Answer from the drawing. Dimensions are ordinates in mm from the lowest x, y and z of the part. A direction names the side the tool comes from. Give positions to 0.01 mm unless a question says otherwise; leave off trailing zeros. Order: outer loops, then holes, each group sorted by start corner. A loop starts at its lowest first (then second) coordinate and runs counter-clockwise, first axis right, second up.
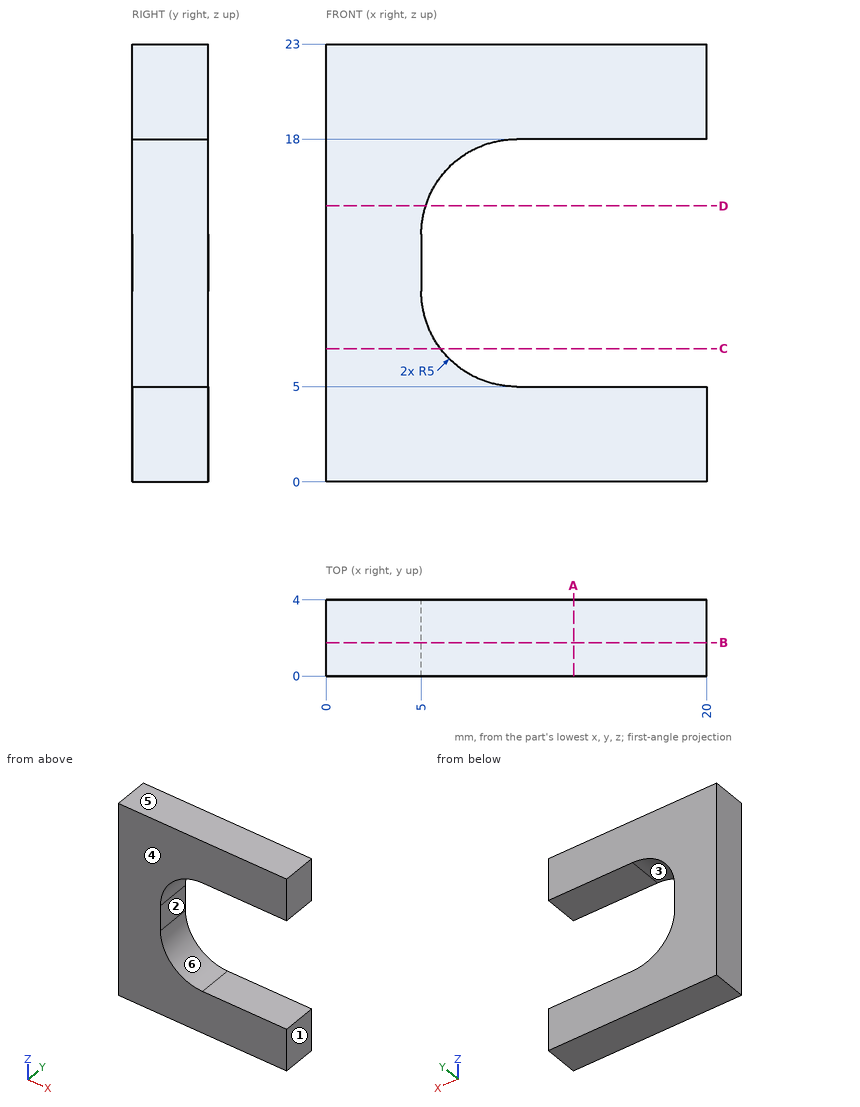
1. The mould has two halves that part along Z. Classify the marked faces 3, 4, 5 and 6: pulls with the +Z half, pulls with the -Z half, needs draft (parallel to the pull), parting line crosses it, or undercut.
Findings below:
face 3: undercut
face 4: needs draft
face 5: pulls with the +Z half
face 6: undercut
2. The part is cut by section B-B (y = 1.75). Write down the section's boundary in (x, z).
Findings below:
outline: (0, 0) - (20, 0) - (20, 5) - (10, 5) arc R5 cw to (5, 10) - (5, 13) arc R5 cw to (10, 18) - (20, 18) - (20, 23) - (0, 23) - close
3. The part is cut by section D-D (z = 14.5). Write down the section's boundary in (x, y).
Findings below:
outline: (0, 0) - (5.23, 0) - (5.23, 4) - (0, 4) - close
4. The part is cut by section C-C (z = 7). Write down the section's boundary in (x, y), then the cut area to 3 significant figures.
Findings below:
outline: (0, 0) - (6, 0) - (6, 4) - (0, 4) - close
area: 24.0 mm2
5. Straight lines are drawn through the part: probe 1 along Z at (x, y) = (13.5, 2.3); probe 2 along Z at (x, y) = (7.5, 0.7); probe 3 along X at (y, z) = (0.85, 11.5). For each, find the intervals that lie inside material, in ascending order.
Findings below:
probe 1: z = 0 to 5, 18 to 23
probe 2: z = 0 to 5.67, 17.33 to 23
probe 3: x = 0 to 5
6. Given P1, Ø1.5, axis at x = 15, y = 0.5, coming from the -Z side; P2, Ø2, axis at y = 0.5, z = 7.5, coming from the +X side; P3, Ø1.5, axis at y = 2.5, z = 11.5, coming from the +X side, each flat-ended and moving along its own axis, determine where each tip first touches the part or whether it passes through.
Findings below:
P1: stops at z = 0
P2: stops at x = 6.43
P3: stops at x = 5
7. Which of the six approach directions +Z, -Z, +X, -X, +Y, -Y give full straight-line access (tool end or side, diameter ignored) to the marked faces 1 and 2?
Findings below:
face 1: +Z, -Z, +X, +Y, -Y
face 2: +X, +Y, -Y
8. The part is cut by section A-A (x = 13). Write down the section's boundary in (y, z).
Findings below:
outline: (0, 0) - (4, 0) - (4, 5) - (0, 5) - close; (0, 18) - (4, 18) - (4, 23) - (0, 23) - close
